```python
from build123d import *

# Parameters (mm, degrees)
SKETCH1_W           = 25.4
SKETCH1_H           = 38.1
SKETCH1_R           = 2.032
BOSS_EXTRUDE1_DEPTH = 3.175
SKETCH2_R           = 2.032
BOSS_EXTRUDE2_DEPTH = 25.4
SKETCH3_W           = 12.7
SKETCH3_H           = 31.75
SKETCH3_W_2         = 3.175
CUT_EXTRUDE1_DEPTH  = 27.181720723
FILLET1_R           = 2.54


with BuildPart() as part:
    # Sketch1 → Boss-Extrude1 (new body)
    with BuildSketch(Plane.XY):
        Rectangle(SKETCH1_W, SKETCH1_H)
        with Locations((-8.466666667, 9.525)):
            Circle(SKETCH1_R, mode=Mode.SUBTRACT)
        with Locations((8.466666667, 9.525)):
            Circle(SKETCH1_R, mode=Mode.SUBTRACT)
        with Locations((-8.466666667, -9.525)):
            Circle(SKETCH1_R, mode=Mode.SUBTRACT)
        with Locations((8.466666667, -9.525)):
            Circle(SKETCH1_R, mode=Mode.SUBTRACT)
    extrude(amount=BOSS_EXTRUDE1_DEPTH)

    # Sketch2 → Boss-Extrude2 (add)
    with BuildSketch(Plane.ZY.offset(12.7)):
        with BuildLine():
            ThreePointArc((15.875, 0), (12.155256121, 8.980256121), (3.175, 12.7))
            Line((3.175, 12.7), (3.175, -19.05))
            Line((3.175, -19.05), (15.875, -19.05))
            Line((15.875, -19.05), (15.875, 0))
        make_face()
        with Locations((11.1125, 0)):
            Circle(SKETCH2_R, mode=Mode.SUBTRACT)
        with Locations((11.1125, -14.2875)):
            Circle(SKETCH2_R, mode=Mode.SUBTRACT)
    extrude(amount=-BOSS_EXTRUDE2_DEPTH)

    # Sketch3 → Cut-Extrude1 (cut, through all)
    with BuildSketch(Plane.XY.offset(3.175)):
        with Locations((0, -3.175)):
            Rectangle(SKETCH3_W, SKETCH3_H)
        with Locations((-14.2875, -3.175)):
            Rectangle(SKETCH3_W_2, SKETCH3_H)
        with Locations((14.2875, -3.175)):
            Rectangle(SKETCH3_W_2, SKETCH3_H)
    extrude(amount=CUT_EXTRUDE1_DEPTH, mode=Mode.SUBTRACT)

    # Fillet1
    fillet1_edges = [part.edges().sort_by_distance(p)[0] for p in [
        (0, 19.05, 3.175),
        (12.7, 15.875, 3.175),
        (9.525, -19.05, 15.875),
        (12.7, -9.525, 15.875),
        (-12.7, -9.525, 15.875),
        (12.7, 8.980256121, 12.155256121),
        (9.525, 12.7, 3.175),
        (-12.7, 8.980256121, 12.155256121),
        (-12.7, 15.875, 3.175),
        (-9.525, 12.7, 3.175),
        (6.35, 8.980256121, 12.155256121),
        (-6.35, 8.980256121, 12.155256121),
        (-9.525, -19.05, 15.875),
        (-6.35, -3.175, 3.175),
        (6.35, -19.05, 9.525),
        (6.35, -3.175, 3.175),
        (6.35, -9.525, 15.875),
        (-6.35, -9.525, 15.875),
        (0, -19.05, 3.175),
        (-6.35, -19.05, 9.525),
    ]]
    fillet(fillet1_edges, radius=FILLET1_R)


solid = part.part
```
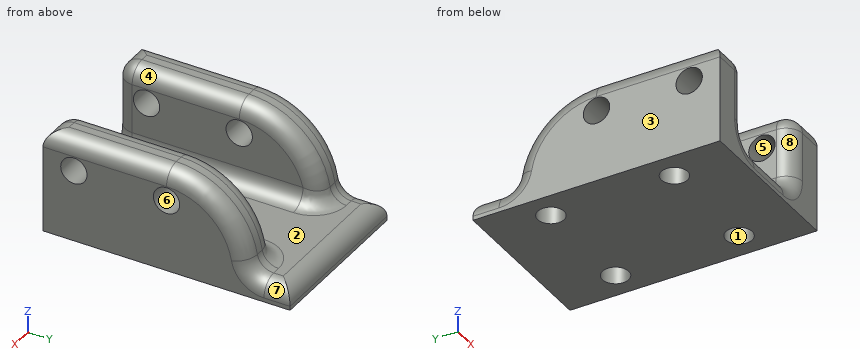
CAD build for the part. Positions are in the model's coordinates, mm. Face numbers are marked on the shaded views. A direction names the side the tool comes from. Round coordinates to 2 decimals unless told otherwise and drop trailing zeros. Loops run counter-clockwise (first coordinate to the right, second up) from the corner with the lowest first, then second, coordinate; pieces in that order, holes last. Notation, with made-up numbers: M 30.5,55 L 47.5,55 A25 cw 47.5,73 Z; hole C 8,-19 d6. An arc over 180 degrees is marked long. Use a Markdown table: item, result. Add a question column.
(1) Drill centre lines: line 1 (X direction, y = 4.5, z = 5.75); line 2 (Y direction, x = 9, z = 10); line 3 (Y direction, x = -10, z = 9.25). Where is each one in solid material? Low to high.
(2) Pull direction X, two halves, no side cores. Call the marked faces 6, 7 and 8: +X half, -X half, draft (parallel to the pull), parting line (faces both ways), or undercut.
(3) Which spindle directions (+Z, -Z, +X, -X, +Y, -Y) get a long thin tool onto all of the face, cutting with end or side? Do the marked faces 1, 2, 3, 4 and 5. Say none if no direction does.
(4) Cut at A-A (y = -13.5). Give the cut face in (x, z) (3 decimals).
(5) Cut at B-B (y = 15.5). Give the cut face in (x, z) (3 decimals), and give its area (3 significant figures).
(6) Flat gauge pins, fed straight in: pin 1 (4.5 mm diameter, centred on y = 0, z = 11.11, fed in from +X); pin 2 (1.2 mm diameter, centred on x = -8, y = -9.5, fed in from -Z) (3 decimals); pin 3 (8 mm diameter, centred on x = -4.5, y = 11.5, fed in from +Z); pin 4 (5.5 mm diameter, centred on x = -8.47, y = 9.52, fed in from +Z). Where does each tip first touch, or does it go through?
Geometry says:
| question | item | result |
|---|---|---|
| 1 | line 1 | x = -12.7 to -6.35, 6.35 to 12.7 |
| 1 | line 2 | y = -19.05 to -15.99, -12.59 to -1.7, 1.7 to 10.71 |
| 1 | line 3 | y = -19.05 to -15.1, -13.48 to -0.81, 0.81 to 11.15 |
| 2 | face 6 | draft |
| 2 | face 7 | +X half |
| 2 | face 8 | undercut |
| 3 | face 1 | -Z |
| 3 | face 2 | +Z, +Y |
| 3 | face 3 | +Z, -Z, -X, +Y, -Y |
| 3 | face 4 | +Z, +Y, -Y |
| 3 | face 5 | +X, -X |
| 4 | outline | M -12.7,0 L 12.7,0 L 12.7,9.239 L 6.35,9.239 L 6.35,5.715 A2.54 cw 3.81,3.175 L -3.81,3.175 A2.54 cw -6.35,5.715 L -6.35,9.239 L -12.7,9.239 Z; M -12.7,12.986 L -6.35,12.986 L -6.35,13.335 A2.54 ccw -8.89,15.875 L -10.16,15.875 A2.54 ccw -12.7,13.335 Z; M 6.35,12.986 L 12.7,12.986 L 12.7,13.335 A2.54 ccw 10.16,15.875 L 8.89,15.875 A2.54 ccw 6.35,13.335 Z |
| 5 | outline | M -12.7,0 L 12.7,0 L 12.7,0.635 A2.54 ccw 10.16,3.175 L -10.16,3.175 A2.54 ccw -12.7,0.635 Z |
| 5 | area | 77.9 mm² |
| 6 | pin 1 | stops at x = 12.7 |
| 6 | pin 2 | stops at z = 3.175 |
| 6 | pin 3 | stops at z = 11.71 |
| 6 | pin 4 | stops at z = 13.91 |
